Could you check a few things on this model? Use its own coordinates, in mm. Face numbers are marked on the shaded views. A direction names the side the tool comes from. Give positions to 0.01 mm unless a question says otherwise; leave off trailing zeros. Loops run counter-clockwise (first coordinate to the right, second up) from the corner with the lowest first, then second, coordinate; pieces in that order, holes last. Notation, with made-up numbers: (-29, 17) - (29, 17) arc R12 cw to (29, 37) - close; hole circle Ø3 at (-20.5, -12.75). An arc over 180 degrees is marked (long way). Use CSV: the item, a comma, the result in double quotes.
from build123d import *

# Parameters (mm, degrees)
SKETCH_1_W           = 100
SKETCH_1_H           = 100
EXTRUDE_1_DEPTH      = 4
SKETCH_2_W           = 4
SKETCH_2_H           = 100
EXTRUDE_2_DEPTH      = 30
SKETCH_3_W           = 70
SKETCH_3_H           = 30
EXTRUDE_3_DEPTH      = 4
SKETCH_4_R           = 2
CUT_EXTRUDE_1_DEPTH  = 128.769323392
SKETCH_5_R           = 1.5
CUT_EXTRUDE_2_DEPTH  = 129.767231857
EXTRUDE_4_DEPTH      = 10
EXTRUDE_4_DEPTH_BACK = 10


with BuildPart() as part:
    # 草图1 → 凸台-拉伸1 (new body)
    with BuildSketch(Plane(origin=(0, 0, 0), x_dir=(0, 0, -1), z_dir=(1, 0, 0))):
        Rectangle(SKETCH_1_W, SKETCH_1_H)
    extrude(amount=EXTRUDE_1_DEPTH)

    # 草图2 → 凸台-拉伸2 (add)
    with BuildSketch(Plane(origin=(4, 0, 0), x_dir=(0, 0, -1), z_dir=(1, 0, 0))):
        with Locations((48, 0)):
            Rectangle(SKETCH_2_W, SKETCH_2_H)
    extrude(amount=EXTRUDE_2_DEPTH)

    # 草图3 → 凸台-拉伸3 (add)
    with BuildSketch(Plane.ZY):
        with Locations((-60, 65)):
            Rectangle(SKETCH_3_W, SKETCH_3_H)
        with Locations((-60, -65)):
            Rectangle(SKETCH_3_W, SKETCH_3_H)
    extrude(amount=-EXTRUDE_3_DEPTH)

    # 草图4 → 切除-拉伸1 (cut, through all)
    with BuildSketch(Plane(origin=(4, 0, 0), x_dir=(0, 0, -1), z_dir=(1, 0, 0))):
        with Locations((75, 70)):
            Circle(SKETCH_4_R)
        with Locations((75, -70)):
            Circle(SKETCH_4_R)
    extrude(amount=-CUT_EXTRUDE_1_DEPTH, mode=Mode.SUBTRACT)

    # 草图5 → 切除-拉伸2 (cut, through all)
    with BuildSketch(Plane.ZY):
        with Locations((46.5, 46.5)):
            Circle(SKETCH_5_R)
        with Locations((-46.5, 46.5)):
            Circle(SKETCH_5_R)
        with Locations((-46.5, -46.5)):
            Circle(SKETCH_5_R)
        with Locations((46.5, -46.5)):
            Circle(SKETCH_5_R)
    extrude(amount=-CUT_EXTRUDE_2_DEPTH, mode=Mode.SUBTRACT)

    # 草图6 → 凸台-拉伸4 (add, two sides: drawn at the far end of the back side and taken through both)
    with BuildSketch(Plane(origin=(0, 0, 0), x_dir=(1, 0, 0), z_dir=(0, 1, 0)).offset(-EXTRUDE_4_DEPTH_BACK)):
        Polygon((4, 31), (19, 46), (4, 46), align=None)
    extrude(amount=EXTRUDE_4_DEPTH + EXTRUDE_4_DEPTH_BACK)


solid = part.part
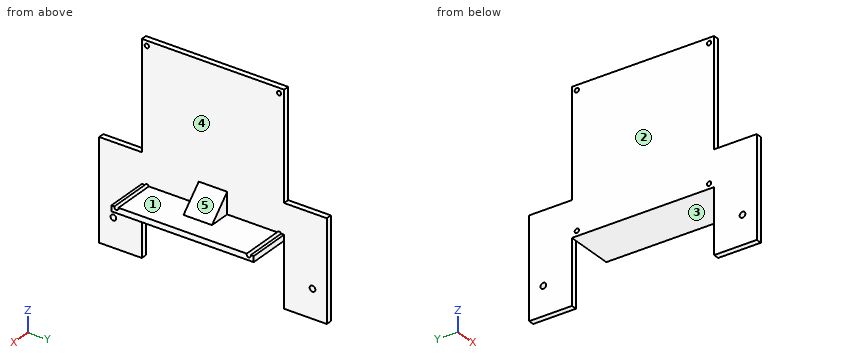
1) I'm going to push flat-ended pins straight in: P1, Ø4.5, axis at x = 2, y = -70, coming from the +Z side; P2, Ø6, axis at x = 28, y = 42.5, coming from the -Z side; P3, Ø1.2, axis at x = 2.5, z = 24.5, coming from the -Y side; P4, Ø3, axis at x = 22, z = -44, coming from the -Y side. Where does each tip first touch, or does it pass through?
Answer below:
P1,"stops at z = -25"
P2,"stops at z = -50"
P3,"stops at y = -50"
P4,"passes through"
2) Suppose I cut it at D-D (z = -43). Please give me the cut outline in (x, y), plus the area to 3 significant figures.
Answer below:
outline,"(0, -80) - (4, -80) - (4, -10) - (16, -10) - (16, 10) - (4, 10) - (4, 80) - (0, 80) - close"
area,"880 mm2"
3) I need wall thicknesses on line 1 along Y through (x, z) = (1.55, 46.5); line 2 along Y through (x, z) = (1.95, -75); line 3 along Z through (x, y) = (7.5, -22). Which ranges of each line are inside material? Lowest first, please.
Answer below:
line 1,"y = -50 to -48, -45 to 45, 48 to 50"
line 2,"y = -80 to -72, -68 to -50, 50 to 68, 72 to 80"
line 3,"z = -50 to -46"
4) We'd pull the mould along Z, two halves only. Please class the marked faces 3, 4 and 5: +Z half, -Z half, draft (parallel to the pull), parting line (faces both ways), or undercut.
Answer below:
face 3,"-Z half"
face 4,"draft"
face 5,"+Z half"
5) Which directions (+Z, -Z, +X, -X, +Y, -Y) give clear straight access to the entire face, cutting with the end or side of a thin tool? Please do the marked faces 1 and 2.
Answer below:
face 1,"+Z, +X"
face 2,"+Z, -Z, -X, +Y, -Y"
6) Suppose I cut it at A-A (y = -70). Please give me the cut outline in (x, z).
Answer below:
outline,"(0, -95) - (4, -95) - (4, -77) - (0, -77) - close; (0, -73) - (4, -73) - (4, -25) - (0, -25) - close"
7) Suppose I cut it at C-C (y = 8). Please give me the cut outline in (x, z), plus the area to 4 significant figures.
Answer below:
outline,"(0, -50) - (34, -50) - (34, -46) - (19, -46) - (4, -31) - (4, 50) - (0, 50) - close"
area,"632.5 mm2"
8) Suppose I cut it at B-B (x = 16.5). Please give me the cut outline in (y, z).
Answer below:
outline,"(-50, -50) - (50, -50) - (50, -46) - (47.91, -46) arc R1.5 cw (long way) to (45.09, -46) - (10, -46) - (10, -43.5) - (-10, -43.5) - (-10, -46) - (-45.09, -46) arc R1.5 cw (long way) to (-47.91, -46) - (-50, -46) - close"
